Autodesk Inventor part; units mm, degrees
ref_plane "作業平面1" through (6, 0, 0) normal (1, 0, 0) x (0, 1, 0)
ref_plane "XZ Plane" through (0, 0, 0) normal (0, 1, 0) x (-1, 0, 0)
ref_plane "XY Plane" through (0, 0, 0) normal (0, 0, 1) x (1, 0, 0)
sketch "スケッチ1" plane through (0, 0, 0) normal (0, 1, 0) x (-1, 0, 0)
  circle A0 centre (0, 0) radius 6
  dimension "d0" = 12
extrude "押し出し1" add sketch "スケッチ1" along normal blind 125
ref_plane "作業平面1" through (6, 0, 0) normal (1, 0, 0) x (0, 1, 0)
sketch "スケッチ2" plane through (6, 0, 0) normal (1, 0, 0) x (0, 1, 0)
  circle A0 centre (62.5, 0) radius 2.5
  line L0 (125, -6) -> (125, 6)
  line L1 (125, 0) -> (0, 0) construction
  line L2 (0, -6) -> (0, 6)
  dimension "d3" = 5
  dimension "d7" = 62.5
extrude "押し出し2" cut sketch "スケッチ2" against normal through all
sketch "スケッチ3" plane through (0, 125, 0) normal (0, 1, 0) x (1, 0, 0)
  circle A0 centre (0, 0) radius 4
  circle A1 centre (0, 0) radius 6
  dimension "d8" = 8
extrude "押し出し3" cut sketch "スケッチ3" against normal blind 10
sketch "スケッチ4" plane through (0, 0, 0) normal (0, -1, 0) x (1, 0, 0)
  circle A0 centre (0, 0) radius 4
  line L0 (3.4641, 2) -> (5.6569, 2)
  line L1 (3.4641, -2) -> (5.6569, -2)
  circle A1 centre (0, 0) radius 6
  line L2 (0, 0) -> (6, 0) construction
  dimension "d11" = 8
  dimension "d12" = 4
extrude "押し出し4" cut sketch "スケッチ4" against normal blind 22 contours A0 | A0 L0 A1 L1 picked at (4.6336, -0.4576)
properties part number "omu_sh_jo_2" material "アルミニウム 6061-AHC"
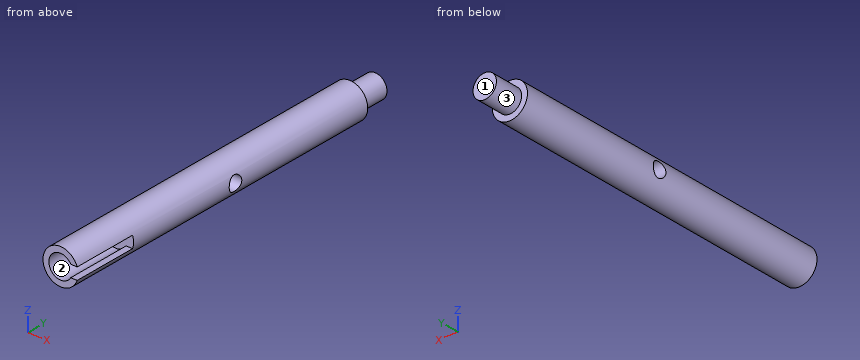
The model under review builds one solid part; all positions refer to its coordinate system, in mm. Face numbers are marked on the shaded views. Coordinates: 2 decimals unless noted, no trailing zeros. Write each loop counter-clockwise with the first axis right and the second up, starting at its lowest first coordinate (ties: lowest second). Pieces come first, ordered by that corner, then holes.
1) Clearance check with flat-ended pins moving along their axes: pin 1 Ø7 at (x, z) = (0, 0) entering from -Y; pin 2 Ø3 at (y, z) = (33.5, -4.5) entering from +X; pin 3 Ø1 at (x, y) = (4.5, 96.5) entering from -Z. State where each tip first meets the part, or that it passes through.
2) The part is to be moulded in two halves that separate along X. For the marked faces 1, 2 and 3, say which applies: pulls with the +X half, pulls with the -X half, needs draft (parallel to the pull), parting line crosses it, or undercut.
3) We need section D-D on y = 62.5. State the section outline as (x, z) points, then the cut area to 3 significant figures.
4) We need section A-A on z = 0. State the section outline as (x, y) points, then the cut area to 3 significant figures.
5) We need section C-C on y = 75.5. State the section outline as (x, z) points.
6) To check wall thickness, follow probe 1 along Z at (x, y) = (0, 62.5); probe 2 along Y at (x, z) = (3, 0); probe 3 along Z at (x, y) = (0, 7.5). State the ranges of each line that lie inside material, in increasing order.
7) We need section B-B on x = 0. State the section outline as (y, z) points.
Answer list:
1. pin 1: stops at y = 22
1. pin 2: stops at x = 5.2
1. pin 3: stops at z = -4.47
2. face 1: needs draft
2. face 2: undercut
2. face 3: parting line crosses it
3. outline: (-5.45, -2.5) arc R6 ccw to (5.45, -2.5) - close; (-5.45, 2.5) - (5.45, 2.5) arc R6 ccw to start
3. area: 54.9 mm2
4. outline: (-6, 0) - (-4, 0) - (-4, 22) - (6, 22) - (6, 60) - (-6, 60) - close; (-6, 65) - (6, 65) - (6, 115) - (4, 115) - (4, 125) - (-4, 125) - (-4, 115) - (-6, 115) - close
4. area: 1,180 mm2
5. outline: circle Ø12 at (0, 0)
6. probe 1: z = -6 to -2.5, 2.5 to 6
6. probe 2: y = 22 to 60, 65 to 125
6. probe 3: z = -6 to -4, 4 to 6
7. outline: (0, -6) - (115, -6) - (115, -4) - (125, -4) - (125, 4) - (115, 4) - (115, 6) - (0, 6) - (0, 4) - (22, 4) - (22, -4) - (0, -4) - close; hole circle Ø5 at (62.5, 0)
